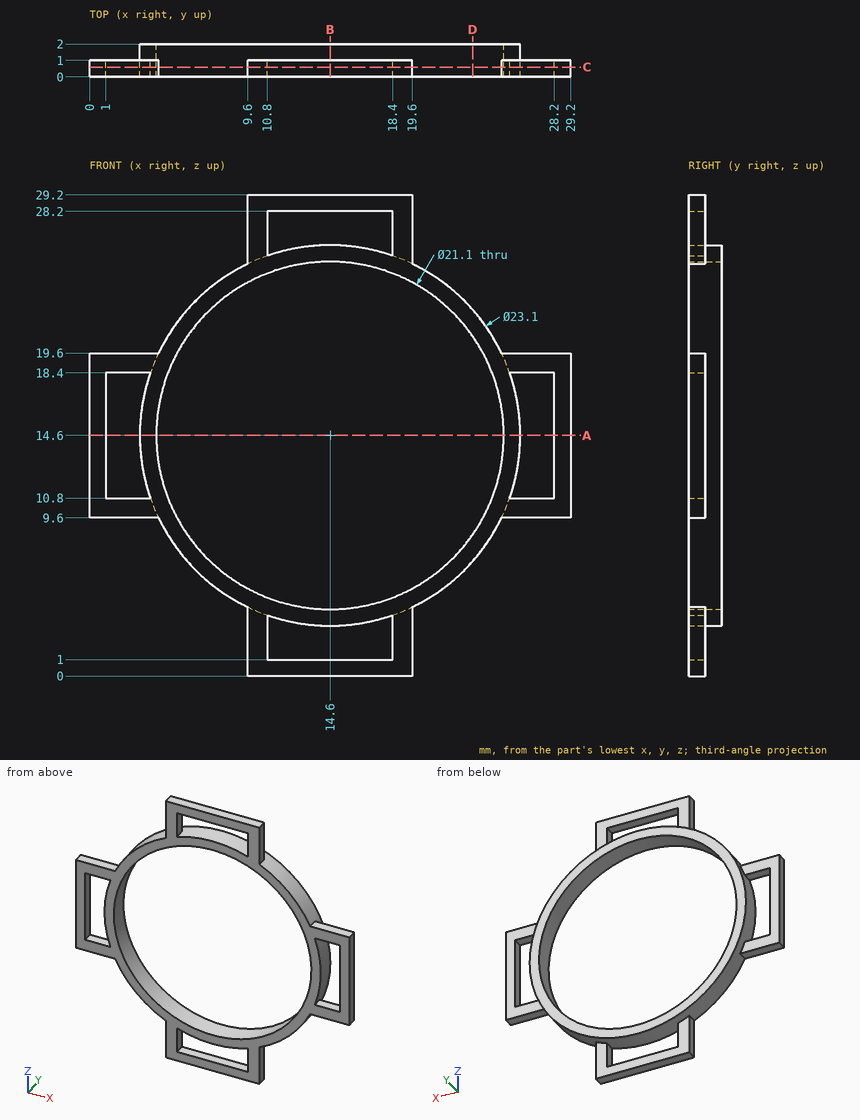
Part print with two shaded views. Sizes in mm from the minimum x, y, z corner. Round coordinates to 2 decimals unless told otherwise and drop trailing zeros. Loops run counter-clockwise (first coordinate to the right, second up) from the corner with the lowest first, then second, coordinate; pieces in that order, holes last.
1. Slice it at D-D (x = 23.25). Give the cut face in (y, z).
Solutions:
outline: (0, 6.95) - (2, 6.95) - (2, 8.56) - (0, 8.56) - close; (0, 20.64) - (2, 20.64) - (2, 22.25) - (0, 22.25) - close
2. Drill centre lines: line 1 along X through (y, z) = (1.2, 14.6); line 2 along X through (y, z) = (0.95, 20); line 3 along Z through (x, y) = (19, 0.4). Where is each one in solid material? Low to high.
Solutions:
line 1: x = 3.05 to 4.05, 25.15 to 26.15
line 2: x = 4.39 to 5.54, 23.66 to 24.81
line 3: z = 0 to 5.01, 24.19 to 29.2
3. Slice it at A-A (z = 14.6). Give the cut face in (x, y), and give its area (3 significant figures).
Solutions:
outline: (0, 0) - (1, 0) - (1, 1) - (0, 1) - close; (3.05, 0) - (4.05, 0) - (4.05, 2) - (3.05, 2) - close; (25.15, 0) - (26.15, 0) - (26.15, 2) - (25.15, 2) - close; (28.2, 0) - (29.2, 0) - (29.2, 1) - (28.2, 1) - close
area: 6.00 mm2
4. Slice it at C-C (y = 0.6). Count the separate pieces of the cut face and the enclosed holes in it, and give its area (3 significant figures).
Solutions:
separate pieces: 1
enclosed holes: 5
area: 138 mm2
5. Slice it at B-B (x = 14.6). Give the cut face in (y, z).
Solutions:
outline: (0, 0) - (1, 0) - (1, 1) - (0, 1) - close; (0, 3.05) - (2, 3.05) - (2, 4.05) - (0, 4.05) - close; (0, 25.15) - (2, 25.15) - (2, 26.15) - (0, 26.15) - close; (0, 28.2) - (1, 28.2) - (1, 29.2) - (0, 29.2) - close
6. Flat gauge pins, fed straight in: pin 1 (0.5 mm diameter, centred on x = 2.5, y = 0.5, fed in from -Z); pin 2 (0.8 mm diameter, centred on y = 0.5, z = 1.5, fed in from -X); pin 3 (0.8 mm diameter, centred on y = 0.5, z = 2, fed in from +X); pin 4 (3 mm diameter, centred on x = 6, z = 13.5, fed in from +Y). Where does each tip first touch, or does it go through?
Solutions:
pin 1: stops at z = 9.6
pin 2: stops at x = 9.6
pin 3: stops at x = 19.6
pin 4: passes through
